Geometry: final body of the model. Coordinates: model frame, mm. A direction names the side the tool comes from. Give positions to 0.01 mm unless a question says otherwise; leave off trailing zeros. Write each loop counter-clockwise with the first axis right and the second up, starting at its lowest first coordinate (ties: lowest second). Pieces come first, ordered by that corner, then holes.
```python
from build123d import *

# Parameters (mm, degrees)
SKETCH1_R           = 12.7
BOSS_EXTRUDE1_DEPTH = 6.35


with BuildPart() as part:
    # Sketch1 → Boss-Extrude1 (new, symmetric)
    # profile 1 of 3: a face of its own
    with BuildSketch(Plane.XY):
        with BuildLine():
            Line((-9.525, 76.2), (-9.525, 136.886260676))
            ThreePointArc((-9.525, 136.886260676), (-18.575269818, 130.663783585), (-24.152491502, 121.202219064))
            ThreePointArc((-24.152491502, 121.202219064), (-24.781960517, 117.271931521), (-25.4, 113.33983048))
            Line((-25.4, 113.33983048), (-25.4, 0))
            ThreePointArc((-25.4, 0), (0, -25.4), (25.4, 0))
            Line((25.4, 0), (25.4, 113.33983048))
            ThreePointArc((25.4, 113.33983048), (24.781960517, 117.271931521), (24.152491502, 121.202219064))
            ThreePointArc((24.152491502, 121.202219064), (18.575269818, 130.663783585), (9.525, 136.886260676))
            Line((9.525, 136.886260676), (9.525, 76.2))
            Line((9.525, 76.2), (-9.525, 76.2))
        make_face()
        Circle(SKETCH1_R, mode=Mode.SUBTRACT)
    # profile 2 of 3: a face of its own
    with BuildSketch(Plane.XY):
        with BuildLine():
            Line((9.525, 177.8), (9.525, 136.886260676))
            ThreePointArc((9.525, 136.886260676), (18.575269818, 130.663783585), (24.152491502, 121.202219064))
            ThreePointArc((24.152491502, 121.202219064), (19.223916585, 149.768263862), (13.691628219, 178.22355426))
            ThreePointArc((13.691628219, 178.22355426), (11.416973573, 179.894050437), (9.525, 177.8))
        make_face()
    # profile 3 of 3: a face of its own
    with BuildSketch(Plane.XY):
        with BuildLine():
            Line((-9.525, 136.886260676), (-9.525, 177.8))
            ThreePointArc((-9.525, 177.8), (-11.416973573, 179.894050437), (-13.691628219, 178.22355426))
            ThreePointArc((-13.691628219, 178.22355426), (-19.223916585, 149.768263862), (-24.152491502, 121.202219064))
            ThreePointArc((-24.152491502, 121.202219064), (-18.575269818, 130.663783585), (-9.525, 136.886260676))
        make_face()
    extrude(amount=BOSS_EXTRUDE1_DEPTH, both=True)


solid = part.part
```
Item 1: Line query: L1, parallel to Y at x = 0, z = 2; L2, parallel to X at y = 1, z = -1.5; L3, parallel to X at y = 96, z = 2.25 (3 decimals). Output: solid intervals per line, ascending.
Found:
L1: y = -25.4 to -12.7, 12.7 to 76.2
L2: x = -25.4 to -12.66, 12.66 to 25.4
L3: x = -25.4 to -9.525, 9.525 to 25.4
Item 2: Pull-direction query (X, two-part tool) for faces 3 (the face through (-0.559, -25.394, 0.089)), 4 (the face through (-25.4, 57, 0)), 5 (the face through (0, 76.2, 0)), 6 (the face through (-9.525, 126, 0)); classes: +X half, -X half, draft (parallel to the pull), parting line (faces both ways), or undercut.
Found:
face 3: parting line
face 4: -X half
face 5: undercut
face 6: undercut
Item 3: Pin query (flat end, axial travel): pin 1 Ø1.5 at (x, z) = (-6, -5) entering from +Y; pin 2 Ø4 at (x, z) = (-5, 1) entering from -Y. Return the tip coordinate at first contact, or that it passes through.
Found:
pin 1: stops at y = 76.2
pin 2: stops at y = -25.22
Item 4: Section B-B, the plane x = 0. Return the cut outline in (y, z), plus the area to 3 significant figures.
Found:
outline: (-25.4, -6.35) - (-12.7, -6.35) - (-12.7, 6.35) - (-25.4, 6.35) - close; (12.7, -6.35) - (76.2, -6.35) - (76.2, 6.35) - (12.7, 6.35) - close
area: 968 mm2
Item 5: Section A-A, the plane z = 3.5. Return the cut outline in (x, y) (1 decimal), plus the area to 3 significant figures.
Found:
outline: (-25.4, 0) arc R25.4 ccw to (25.4, 0) - (25.4, 113.3) arc R1369.1 ccw to (24.2, 121.2) arc R1369.1 ccw to (13.7, 178.2) arc R2.1 ccw to (9.5, 177.8) - (9.5, 76.2) - (-9.5, 76.2) - (-9.5, 177.8) arc R2.1 ccw to (-13.7, 178.2) arc R1369.1 ccw to (-24.2, 121.2) arc R1369.1 ccw to (-25.4, 113.3) - close; hole circle Ø25.4 at (0, 0)
area: 6,900 mm2
Item 6: Reachability of faces 1 (the face through (25.4, 56, 0)), 2 (the face through (9.525, 128, 0)) from +Z, -Z, +X, -X, +Y, -Y: full face, straight path, thin tool, end or side. Return the list, or none.
Found:
face 1: +Z, -Z, +X, +Y, -Y
face 2: +Z, -Z, +Y
Item 7: Section C-C, the plane y = 164. Return the cut outline in (x, z) (3 decimals).
Found:
outline: (-16.535, -6.35) - (-9.525, -6.35) - (-9.525, 6.35) - (-16.535, 6.35) - close; (9.525, -6.35) - (16.535, -6.35) - (16.535, 6.35) - (9.525, 6.35) - close
